For this review, take the finished solid that the model builds, in its own axes (mm). A direction names the side the tool comes from. Give positions to 0.01 mm unless a question says otherwise; leave off trailing zeros. Loops run counter-clockwise (first coordinate to the right, second up) from the corner with the lowest first, then second, coordinate; pieces in that order, holes last.
```python
from build123d import *

# Parameters (mm, degrees)
F3_R     = 12.5
F4_DEPTH = 10
F6_DEPTH = 30
F7_R     = 5


with BuildPart() as f2:
    # F2: sweep along a path in F1
    with BuildLine(Plane.XZ) as f2_path:
        Line((0, 0), (250, 0))
    # F0 (on Right) → F2 (sweep)
    with BuildSketch(Plane.YZ):
        Polygon((8, 150), (0, 150), (-8, 150), (-8, 180), (-33, 180), (-33, -180), (-8, -180), (-8, -150), (0, -150), (8, -150), (8, -180), (33, -180), (33, 180), (8, 180), align=None)
    sweep(path=f2_path.line)

    # F3 (on face) → F4 (cut)
    with BuildSketch(Plane.XZ.offset(33)):
        with Locations((220, 150)):
            Circle(F3_R)
    extrude(amount=-F4_DEPTH, mode=Mode.SUBTRACT)

    # F5 (on face) → F6 (cut)
    with BuildSketch(Plane.YZ.offset(250)):
        Polygon((8, 150), (0, 150), (-8, 150), (-8, -150), (0, -150), (8, -150), align=None)
    extrude(amount=-F6_DEPTH, mode=Mode.SUBTRACT)

    # F7
    f7_edges = [f2.edges().sort_by_distance(p)[0] for p in [
        (110, 8, 150),
        (220, 0, 150),
        (110, -8, 150),
        (0, 0, 150),
        (110, -8, -150),
        (220, 0, -150),
        (110, 8, -150),
        (0, 0, -150),
        (125, 33, 180),
        (0, 20.5, 180),
        (125, 8, 180),
        (250, 20.5, 180),
        (125, -8, 180),
        (0, -20.5, 180),
        (125, -33, 180),
        (250, -20.5, 180),
        (125, 8, -180),
        (0, 20.5, -180),
        (125, 33, -180),
        (250, 20.5, -180),
        (125, -33, -180),
        (0, -20.5, -180),
        (125, -8, -180),
        (250, -20.5, -180),
        (0, -8, 165),
        (0, -8, -165),
        (0, 8, -165),
        (0, 8, 165),
        (250, 8, 0),
        (250, 33, 0),
        (250, -8, 0),
        (250, -33, 0),
        (220, -8, 0),
        (220, 8, 0),
    ]]
    fillet(f7_edges, radius=F7_R)


solid = f2.part
```
Q1. Machinability: for faces 1 (the flat face through (250, 20, -2)), 2 (the flat face through (220, -23, 150)), 3 (the flat face through (232, -8, -27)), which of the approach directions +Z, -Z, +X, -X, +Y, -Y give a long, thin tool a straight path to every point of the face, cutting with its end or side? Answer none if there is none.
Answers:
face 1: +Z, -Z, +X, +Y, -Y
face 2: -Y
face 3: +X
Q2. Consider section A-A on z = 96. Give the boundary of the cut face in (x, y).
Answers:
outline: (0, -33) - (245, -33) arc R5 ccw to (250, -28) - (250, -13) arc R5 ccw to (245, -8) - (225, -8) arc R5 cw to (220, -3) - (220, 3) arc R5 cw to (225, 8) - (245, 8) arc R5 ccw to (250, 13) - (250, 28) arc R5 ccw to (245, 33) - (0, 33) - close
Q3. Consider section B-B on x = 39.5. Give the boundary of the cut face in (y, z), plus the area to 3 significant figures.
Answers:
outline: (-33, -175) arc R5 ccw to (-28, -180) - (-13, -180) arc R5 ccw to (-8, -175) - (-8, -155) arc R5 cw to (-3, -150) - (3, -150) arc R5 cw to (8, -155) - (8, -175) arc R5 ccw to (13, -180) - (28, -180) arc R5 ccw to (33, -175) - (33, 175) arc R5 ccw to (28, 180) - (13, 180) arc R5 ccw to (8, 175) - (8, 155) arc R5 cw to (3, 150) - (-3, 150) arc R5 cw to (-8, 155) - (-8, 175) arc R5 ccw to (-13, 180) - (-28, 180) arc R5 ccw to (-33, 175) - close
area: 22,800 mm2
Q4. For pin 1 Ø3 at (y, z) = (0.5, 21.5) entering from +X; pin 2 Ø1.8 at (x, y) = (95, -0.5) entering from +Z; pin 3 Ø1.8 at (x, y) = (69.5, 0.5) entering from -Z, all flat-tipped, find the tip position at first contact; note any pin that passes through.
Answers:
pin 1: stops at x = 220
pin 2: stops at z = 150
pin 3: stops at z = -150
Q5. For probe 1 along Y at (x, z) = (29, -164); probe 2 along Z at (x, y) = (220, -27.75); probe 3 along X at (y, z) = (-27.5, 152.5), list the stretches that pass through material, from the lowest coordinate up.
Answers:
probe 1: y = -33 to -8, 8 to 33
probe 2: z = -180 to 137.5, 162.5 to 180
probe 3: x = 0 to 207.75, 232.25 to 250
Q6. Mouldability with a two-part tool opening along Z and no side actions: class faces 4 (the flat face through (127, -21, -180)), 5 (the cylindrical face through (226.72, -28.07, 160.54)), 6 (the flat face through (124, 33, -2)) as +Z half, -Z half, draft (parallel to the pull), parting line (faces both ways), or undercut.
Answers:
face 4: -Z half
face 5: undercut
face 6: draft
